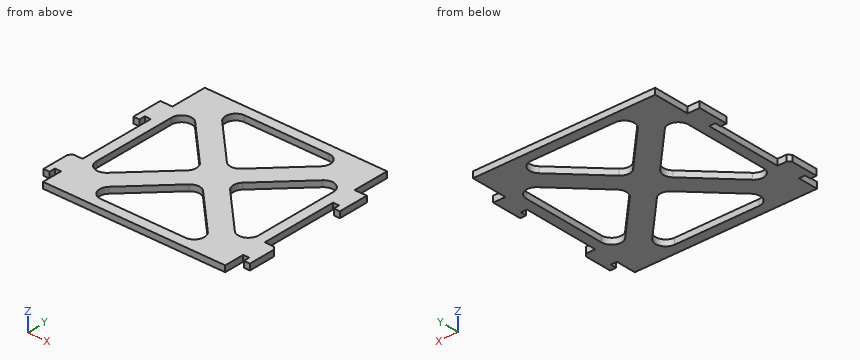
```python
from build123d import *

# Parameters (mm, degrees)
F0_W     = 90
F0_H     = 90
F1_DEPTH = 3
F3_DEPTH = 3
F4_SIZE  = 1.5


with BuildPart() as f1:
    # F0 (on Top) → F1 (new body)
    with BuildSketch(Plane.XY):
        Rectangle(F0_W, F0_H)
        with BuildLine():
            Line((3.535534, -10.606602), (24.393397, -31.464465))
            ThreePointArc((24.393397, -31.464465), (25.477261, -36.913416), (20.857863, -39.999999))
            Line((20.857863, -39.999999), (-20.857864, -39.999999))
            ThreePointArc((-20.857864, -39.999999), (-25.477261, -36.913416), (-24.393398, -31.464465))
            Line((-24.393398, -31.464465), (-3.535534, -10.606602))
            ThreePointArc((-3.535534, -10.606602), (0, -9.142136), (3.535534, -10.606602))
        make_face(mode=Mode.SUBTRACT)
        with BuildLine():
            ThreePointArc((-40, 20.857864), (-36.913417, 25.477262), (-31.464466, 24.393398))
            Line((-31.464466, 24.393398), (-10.606602, 3.535534))
            ThreePointArc((-10.606602, 3.535534), (-9.142136, 0), (-10.606602, -3.535534))
            Line((-10.606602, -3.535534), (-31.464466, -24.393398))
            ThreePointArc((-31.464466, -24.393398), (-36.913417, -25.477262), (-40, -20.857864))
            Line((-40, -20.857864), (-40, 20.857864))
        make_face(mode=Mode.SUBTRACT)
        with BuildLine():
            ThreePointArc((20.857863, 39.999999), (25.477261, 36.913416), (24.393397, 31.464465))
            Line((24.393397, 31.464465), (3.535534, 10.606602))
            ThreePointArc((3.535534, 10.606602), (0, 9.142136), (-3.535534, 10.606602))
            Line((-3.535534, 10.606602), (-24.393398, 31.464465))
            ThreePointArc((-24.393398, 31.464465), (-25.477261, 36.913416), (-20.857864, 39.999999))
            Line((-20.857864, 39.999999), (20.857863, 39.999999))
        make_face(mode=Mode.SUBTRACT)
        with BuildLine():
            Line((10.606602, 3.535534), (31.464466, 24.393398))
            ThreePointArc((31.464466, 24.393398), (36.913417, 25.477262), (40, 20.857864))
            Line((40, 20.857864), (40, -20.857864))
            ThreePointArc((40, -20.857864), (36.913417, -25.477262), (31.464466, -24.393398))
            Line((31.464466, -24.393398), (10.606602, -3.535534))
            ThreePointArc((10.606602, -3.535534), (9.142136, 0), (10.606602, 3.535534))
        make_face(mode=Mode.SUBTRACT)
    extrude(amount=F1_DEPTH)

    # F2 (on face) → F3 (join, through all)
    with BuildSketch(Plane(origin=(0, 0, 0), x_dir=(1, 0, 0), z_dir=(0, 0, -1))):
        Polygon((45, -15), (45, -27), (51, -27), (51, -12), (48, -12), (48, -15), align=None)
        Polygon((45, 35), (45, 23), (51, 23), (51, 38), (48, 38), (48, 35), align=None)
        Polygon((-45, -15), (-48, -15), (-48, -12), (-51, -12), (-51, -27), (-45, -27), align=None)
        Polygon((-45, 23), (-45, 35), (-48, 35), (-48, 38), (-51, 38), (-51, 23), align=None)
    extrude(amount=-F3_DEPTH)

    # F4
    f4_edges = [f1.edges().sort_by_distance(p)[0] for p in [
        (-51, -23, 1.5),
        (51, -23, 1.5),
    ]]
    chamfer(f4_edges, length=F4_SIZE)


solid = f1.part
```
Input: part model. Units: mm. Frame: model coordinates. Round coordinates to 2 decimals unless told otherwise and drop trailing zeros. Order: outer loops, then holes, each group sorted by start corner. A loop starts at its lowest first (then second) coordinate and runs counter-clockwise, first axis right, second up. Notation, with made-up numbers: (15.25, 19.5) - (24.25, 19.5) arc R7 cw to (24.25, 26.5) - close; hole circle Ø8 at (67.25, 41). An arc over 180 degrees is marked (long way). One line per question, with ' | ' between items. Start each with the question number.
1) Cut plane D-D, the plane z = 1.65. Give the number of separate pieces and of enclosed holes in the cut face, then the cut area to 3 significant figures.
2) Cut plane B-B, the plane y = -33. Return the cut outline in (x, z), then the cut area to 3 significant figures.
3) Cut plane C-C, the plane x = -15. Return the cut outline in (y, z), then the cut area to 3 significant figures.
4) Ray query, probe 1 along X at (y, z) = (-34.5, 0.25); probe 2 along Y at (x, z) = (-25, 1.1); probe 3 along Y at (x, z) = (-17, 0.4). Return the intervals inside material, ascending.
5) Contact query for flat-ended pins moving along their axis: P1, Ø1.5, axis at y = 35, z = 2, coming from the +X side; P2, Ø10, axis at x = 14, y = -16.5, coming from the -Z side; P3, Ø0.9, axis at x = 49, z = 1.5, coming from the +Y side; P4, Ø1.5, axis at x = 50, z = 1, coming from the -Y side. Output: stop coordinate, or through.
6) Cut plane A-A, the plane x = 5.5. Return the cut outline in (y, z).
Worked out:
1) separate pieces: 1 | enclosed holes: 4 | area: 4,350 mm^2
2) outline: (-51, 0) - (-25.44, 0) - (-25.44, 3) - (-51, 3) - close; (25.44, 0) - (51, 0) - (51, 3) - (25.44, 3) - close | area: 153 mm^2
3) outline: (-45, 0) - (-40, 0) - (-40, 3) - (-45, 3) - close; (-22.07, 0) - (-7.93, 0) - (-7.93, 3) - (-22.07, 3) - close; (7.93, 0) - (22.07, 0) - (22.07, 3) - (7.93, 3) - close; (40, 0) - (45, 0) - (45, 3) - (40, 3) - close | area: 115 mm^2
4) probe 1: x = -51 to -25.83, 25.83 to 51 | probe 2: y = -45 to -37.8, -32.2 to -17.93, 17.93 to 32.2, 37.8 to 45 | probe 3: y = -45 to -40, -24.07 to -9.93, 9.93 to 24.07, 40 to 45
5) P1: stops at x = 45 | P2: stops at z = 0 | P3: stops at y = 27 | P4: stops at y = -38
6) outline: (-45, 0) - (-40, 0) - (-40, 3) - (-45, 3) - close; (-12.57, 0) - (12.57, 0) - (12.57, 3) - (-12.57, 3) - close; (40, 0) - (45, 0) - (45, 3) - (40, 3) - close
